```python
from build123d import *

# Parameters (mm, degrees)
F4_DEPTH = 15
F5_R     = 85
F5_R_2   = 80
F6_DEPTH = 15
F7_W     = 10
F7_H     = 10
F8_DEPTH = 3


with BuildPart() as f4:
    # F3 (on Top) → F4 (new body)
    with BuildSketch(Plane.XY):
        Polygon((24.3933982822, 50), (-24.3933982822, 50), (-35, 39.3933982822), (-35, 10.6066017178), (-24.3933982822, 0), (-10, 0), (-10, -30), (-20.2512626585, -30), (-25, -25.2512626585), (-25, -15), (-35, -15), (-35, -29.3933982822), (-24.3933982822, -40), (-10, -40), (-10, -50), (-20, -50), (-20, -60), (10, -60), (10, -50), (0, -50), (0, -40), (24.3933982822, -40), (35, -29.3933982822), (35, -0.6066017178), (24.3933982822, 10), (0, 10), (0, 12.3223304703), (0, 20), (35, 20), (35, 10), (45, 10), (45, 30), (-20, 30), (-20, 20), (-10, 20), (-10, 18.4070525334), (-10, 10), (-20.2512626585, 10), (-25, 14.7487373415), (-25, 18.8908729653), (-25, 35.2512626585), (-20.2512626585, 40), (20.2512626585, 40), (25, 35.2512626585), (35, 35.2512626585), (35, 39.3933982822), align=None)
        Polygon((20.2512626585, 0), (25, -4.7487373415), (25, -25.2512626585), (20.2512626585, -30), (0, -30), (0, -20), (15, -20), (15, -10), (0, -10), (0, 0), align=None, mode=Mode.SUBTRACT)
    extrude(amount=F4_DEPTH)



with BuildPart() as f6:
    # F5 (on Top) → F6 (new body)
    with BuildSketch(Plane.XY):
        Circle(F5_R)
        Circle(F5_R_2, mode=Mode.SUBTRACT)
    extrude(amount=F6_DEPTH)


with BuildPart() as f4_1:
    add(f4.part)

    add(f6.part)  # F8 merges F6
    # F7 (on face) → F8 (join)
    with BuildSketch(Plane.XY.offset(15)):
        Rectangle(F7_W, F7_H)
        with BuildLine():
            Line((79.8435971134, 5), (5, 5))
            Line((5, 5), (5, -5))
            Line((5, -5), (79.8435971134, -5))
            ThreePointArc((79.8435971134, -5), (79.9608897183, -2.5012227941), (80, 0))
            ThreePointArc((80, 0), (79.9608897183, 2.5012227941), (79.8435971134, 5))
        make_face()
        with BuildLine():
            Line((-5, 79.8435971134), (-5, 5))
            Line((-5, 5), (5, 5))
            Line((5, 5), (5, 79.8435971134))
            ThreePointArc((5, 79.8435971134), (0, 80), (-5, 79.8435971134))
        make_face()
        with BuildLine():
            Line((-5, 5), (-79.8435971134, 5))
            ThreePointArc((-79.8435971134, 5), (-80, 0), (-79.8435971134, -5))
            Line((-79.8435971134, -5), (-5, -5))
            Line((-5, -5), (-5, 5))
        make_face()
        with BuildLine():
            Line((5, -5), (-5, -5))
            Line((-5, -5), (-5, -79.8435971134))
            ThreePointArc((-5, -79.8435971134), (0, -80), (5, -79.8435971134))
            Line((5, -79.8435971134), (5, -5))
        make_face()
    extrude(amount=-F8_DEPTH)


solid = f4_1.part
```
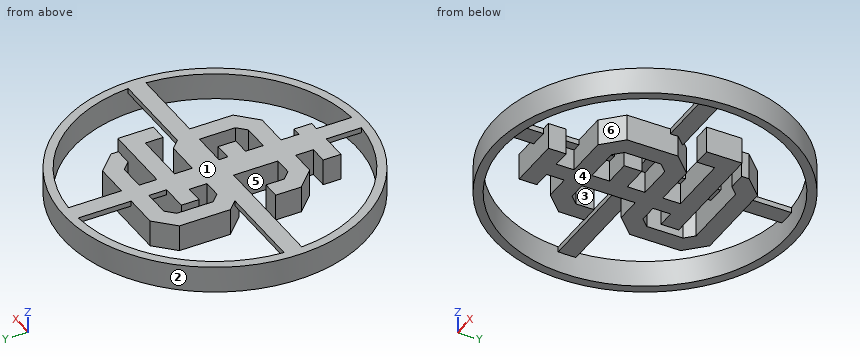
Can you work these out from the model? Positions are in its coordinate system, mm. Face numbers are marked on the shaded views. A direction names the side the tool comes from. Round coordinates to 2 decimals unless told otherwise and drop trailing zeros. Loops run counter-clockwise (first coordinate to the right, second up) from the corner with the lowest first, then second, coordinate; pieces in that order, holes last. Notation, with made-up numbers: M 39,-34.75 L 53,-34.75 A38 cw 53,4.25 Z; hole C -31.5,-5 d5. An arc over 180 degrees is marked long. Answer in a Markdown table with one row per item.
1. If we section it at C-C, the plane y = -18: Please give me the cut outline in (x, z), plus the area to 3 significant figures.
Established:
| item | result |
|---|---|
| outline | M -83.07,0 L -77.95,0 L -77.95,15 L -83.07,15 Z; M -35,0 L -25,0 L -25,15 L -35,15 Z; M -10,0 L 15,0 L 15,15 L -10,15 Z; M 25,0 L 35,0 L 35,15 L 25,15 Z; M 77.95,0 L 83.07,0 L 83.07,15 L 77.95,15 Z |
| area | 829 mm² |
2. Please list where these lines run through material, in increasing order: line 1 (Y direction, x = -22.5, z = 3.25); line 2 (X direction, y = 14.5, z = 8); line 3 (Y direction, x = -54.5, z = 13.25). Write a range as from..to.
Established:
| item | result |
|---|---|
| line 1 | -81.97..-76.77, -40..-27.75, 0..12.25, 37.75..50, 76.77..81.97 |
| line 2 | -83.75..-78.67, -35..-24.75, -10..0, 35..45, 78.67..83.75 |
| line 3 | -65.23..-58.56, -5..5, 58.56..65.23 |
3. If we section it at A-A, the plane x = 75: Please give me the cut outline in (y, z), plus the area to 3 significant figures.
Established:
| item | result |
|---|---|
| outline | M -40,0 L -27.84,0 L -27.84,15 L -40,15 Z; M -5,12 L 5,12 L 5,15 L -5,15 Z; M 27.84,0 L 40,0 L 40,15 L 27.84,15 Z |
| area | 395 mm² |
4. I'm going to push flat-ended pins straight in: pin 1 Ø5 at (y, z) = (-56, 9.5) entering from +X; pin 2 Ø6 at (x, z) = (55.5, 6) entering from -Y; pin 3 Ø3 at (x, z) = (16.5, 11) entering from +Y. Where does each tip first touch, or does it pass through?
Established:
| item | result |
|---|---|
| pin 1 | x = 66.05 |
| pin 2 | y = -66.85 |
| pin 3 | y = 83.67 |
5. On a 3-axis mill with a long thin cutter (end or side, diameter ignored), from which of +Z, -Z, +X, -X, +Y, -Y can I reach the whole of each face in a straight line? I mean the marked faces 4, 5 and 6. Say none if no direction works.
Established:
| item | result |
|---|---|
| face 4 | -Z, +X, -X, +Y, -Y |
| face 5 | -Z |
| face 6 | +Z, -Z |
6. If we section it at D-D, the plane x = 31.5: Please give me the cut outline in (y, z), plus the area to 3 significant figures.
Established:
| item | result |
|---|---|
| outline | M -78.95,0 L -73.54,0 L -73.54,15 L -78.95,15 Z; M -32.89,0 L 2.89,0 L 2.89,12 L 5,12 L 5,15 L -32.89,15 Z; M 20,0 L 30,0 L 30,15 L 20,15 Z; M 35.25,0 L 42.89,0 L 42.89,15 L 35.25,15 Z; M 73.54,0 L 78.95,0 L 78.95,15 L 73.54,15 Z |
| area | 970 mm² |
7. Thinking about a two-plate mould opening in X: for the marked faces 1, 2 and 3, which applies, pulls with the +X half, pulls with the -X half, needs draft (parallel to the pull), parting line crosses it, or undercut?
Established:
| item | result |
|---|---|
| face 1 | needs draft |
| face 2 | parting line crosses it |
| face 3 | undercut |
8. If we section it at B-B, the plane z = 9.25: Give the number of separate pieces and of enclosed holes in the cut face, plus the area to 3 significant figures.
Established:
| item | result |
|---|---|
| separate pieces | 2 |
| enclosed holes | 2 |
| area | 6,920 mm² |
